Work out the finished part from the listing and answer in its coordinate system (mm). A direction names the side the tool comes from. Give positions to 0.01 mm unless a question says otherwise; leave off trailing zeros. Order: outer loops, then holes, each group sorted by start corner. A loop starts at its lowest first (then second) coordinate and runs counter-clockwise, first axis right, second up.
Autodesk Inventor part; units mm, degrees
ref_plane "Work Plane1" through (29, 0, 0) normal (0, -1, 0) x (1, 0, 0)
ref_plane "YZ Plane" through (0, 0, 0) normal (1, 0, 0) x (0, 1, 0)
ref_plane "XZ Plane" through (0, 0, 0) normal (0, 1, 0) x (-1, 0, 0)
sketch "Эскиз1" plane through (0, 0, 0) normal (0, 0, 1) x (1, 0, 0)
  line L0 (-0.0667, 0) -> (8, 0)
  line L1 (8, 0) -> (8, 2)
  line L2 (8, 2) -> (1.4, 2)
  line L3 (1.4, 2) -> (0.9705, 2)
  line L4 (0.9705, 2) -> (0, 2)
  line L5 (0, 2) -> (0, 3.8)
  line L6 (0, 3.8) -> (-2.2, 3.8)
  line L7 (-2.2, 3.8) -> (-2.2, 1.4434)
  line L8 (-2.2, 1.4434) -> (-0.9, 1.4434)
  line L9 (-0.9, 1.4434) -> (-0.0667, 0)
  line L10 (-4.24, 0) -> (10.04, 0)
  line L11 (0, -0.76) -> (0, 4.56)
  line L12 (1.4, 2) -> (0, 2) construction
  dimension "d1" = 6.6
  dimension "d2" = 0.4295
  dimension "d3" = 2.2
  dimension "d4" = 1.3
  dimension "d5" = 60
  dimension "d6" = 4
  dimension "d7" = 4
  dimension "d8" = 2.8868
  dimension "d9" = 7.6
  dimension "d26" = 8
revolve "Базовый элемент" add sketch "Эскиз1" angle 360 about axis through (-0.0667, 0, 0) along (1, 0, 0)
sketch "Эскиз2" plane through (-2.2, 0, 0) normal (-1, 0, 0) x (0, 0, 1)
  circle A0 centre (0, 0) radius 1.4434
  line L0 (0, -5.32) -> (0, 5.32)
  line L1 (-5.32, 0) -> (5.32, 0)
  line L2 (1.4434, 0) -> (0.7217, -1.25)
  line L3 (0.7217, -1.25) -> (-0.7217, -1.25)
  line L4 (-0.7217, -1.25) -> (-1.4434, 0)
  line L5 (-1.4434, 0) -> (-0.7217, 1.25)
  line L6 (-0.7217, 1.25) -> (0.7217, 1.25)
  line L7 (0.7217, 1.25) -> (1.4434, 0)
  point P0 (0, 0)
extrude "Паз" add sketch "Эскиз2" against normal up to next contours L7 A0 | A0 L2 | L6 L0 A0 | A0 L0 L3 | L0 L6 A0 | A0 L3 L0 | L4 A0 | A0 L5
fillet "Сопряжение1" radius 1.87 1 edges at (-2.2, -3.8, 0)
thread "Резьба"
chamfer "Фаска1" distance 0.4294 distance2 0.4294 1 edges at (8, -2, 0) measured on face at (8, 0.556, 0.0273)
ref_plane "Work Plane1" through (29, 0, 0) normal (0, -1, 0) x (1, 0, 0)
fillet "Fillet2" radius 0.1 1 edges at (0, -2, 0)
equation "\"d1\" = GEL"
equation "\"d3\" = KOH"
equation "\"d4\" = INTI"
equation "\"d6\" = GD"
equation "\"d7\" = BDM"
equation "\"d8\" = 1.1547 * SW"
equation "\"d9\" = KOD"
equation "\"d26\" = NLG"
equation "\"d30\" = R"
equation "\"d17\" = RR"
equation "\"d13\" = GEL"
equation "\"d15\" = -0.5 * SPD + 0.5 * GD"
equation "\"d16\" = GUL"
equation "\"GD\" = NND"
equation "\"NLG\" = 8"
equation "\"GEL\" = 6.6"
equation "\"KOD\" = 7.6"
equation "\"KOH\" = 2.2"
equation "\"INTI\" = 1.3"
equation "\"GAL\" = 0.61345 * PTC"
equation "\"GUL\" = 0.61345 * PTC"
equation "\"BDM\" = NND"
equation "\"SW\" = 2.5"
equation "\"RR\" = 1.87"
equation "\"SPD\" = 3.14117"
equation "\"R\" = 0.1"
equation "\"TOA\" = 30deg"
equation "\"GD1\" = THREADDIA - 1.2269 * PTC"
equation "\"THREADDIA\" = 4"
equation "\"PTC\" = 0.7"
equation "\"NND\" = 4"
equation "\"E0\" = 2.87"
properties part number "JIS B 1174 - M4 x 8" material "Сталь, мягкая"
1. Which of the six approach directions +Z, -Z, +X, -X, +Y, -Y give full straight-line access (tool end or side, diameter ignored) to faces 1 (the face through (8, 0, 0)), 2 (the face through (-1.504, 0.616, -1.088))?
Findings below:
face 1: +Z, -Z, +X, +Y, -Y
face 2: -X
2. The mould has two halves that part along Y. Classify faces 3 (the face through (0, 2, -2)), 4 (the face through (-0.12, 0.09, -0.03)), 5 (the face through (4, 0, 2)), 6 (the face through (-1.5, 0.63, 1.08)): pulls with the +Y half, pulls with the -Y half, needs draft (parallel to the pull), parting line crosses it, or undercut.
Findings below:
face 3: needs draft
face 4: undercut
face 5: parting line crosses it
face 6: undercut
3. Straight lines are drawn through the part: probe 1 along Z at (x, y) = (7.25, 0); probe 2 along Z at (x, y) = (6.75, 1.75); probe 3 along Y at (x, z) = (2.5, 1.25). For each, find the intervals that lie inside material, in ascending order.
Findings below:
probe 1: z = -2 to 2
probe 2: z = -0.97 to 0.97
probe 3: y = -1.56 to 1.56
4. Given P1, Ø1.5, axis at x = 0.5, z = 0.5, coming from the -Y side; P2, Ø1.1, axis at x = -1.5, z = 0, coming from the -Y side; P3, Ø1.5, axis at x = -0.5, y = 1.5, coming from the -Z side; P4, Ø1.1, axis at x = -1.5, z = 0, coming from the +Y side, each flat-ended and moving along its own axis, determine where each tip first touches the part or whether it passes through.
Findings below:
P1: stops at y = -3.8
P2: stops at y = -3.69
P3: stops at z = -3.72
P4: stops at y = 3.69
5. The part is cut by section A-A (x = 5.25). Write down the section's boundary in (y, z).
Findings below:
outline: circle Ø4 at (0, 0)
